```python
from build123d import *

# Parameters (mm, degrees)
CUT_EXTRUDE1_DEPTH = 10
FILLET1_R          = 10
SKETCH5_R          = 2
CUT_EXTRUDE2_DEPTH = 10


with BuildPart() as part:
    # Sketch3 → Revolve1 (revolve)
    with BuildSketch(Plane(origin=(0, 0, 0), x_dir=(0, 0, -1), z_dir=(1, 0, 0))):
        Polygon((0, 12), (7, 12), (7, 8), (17, 8), (17, 12), (24, 12), (24, 35), (19, 35), (19, 17), (0, 17), align=None)
    revolve(axis=Axis((0, 0, 0), (0, 0, -1)))

    # Sketch4 → Cut-Extrude1 (cut)
    with BuildSketch(Plane.XY.offset(-19)):
        with BuildLine():
            ThreePointArc((35, 0), (32.335783638, 13.393920133), (24.748737342, 24.748737342))
            Line((24.748737342, 24.748737342), (24.748737342, -24.748737342))
            ThreePointArc((24.748737342, -24.748737342), (32.335783638, -13.393920133), (35, 0))
        make_face()
        with BuildLine():
            ThreePointArc((24.748737342, 24.748737342), (0, 35), (-24.748737342, 24.748737342))
            Line((-24.748737342, 24.748737342), (24.748737342, 24.748737342))
        make_face()
        with BuildLine():
            Line((-24.748737342, -24.748737342), (-24.748737342, 24.748737342))
            ThreePointArc((-24.748737342, 24.748737342), (-35, 0), (-24.748737342, -24.748737342))
        make_face()
        with BuildLine():
            Line((24.748737342, -24.748737342), (-24.748737342, -24.748737342))
            ThreePointArc((-24.748737342, -24.748737342), (0, -35), (24.748737342, -24.748737342))
        make_face()
    extrude(amount=-CUT_EXTRUDE1_DEPTH, mode=Mode.SUBTRACT)

    # Fillet1
    fillet1_edges = [part.edges().sort_by_distance(p)[0] for p in [
        (24.748737342, 24.748737342, -21.5),
        (24.748737342, -24.748737342, -21.5),
        (-24.748737342, 24.748737342, -21.5),
        (-24.748737342, -24.748737342, -21.5),
    ]]
    fillet(fillet1_edges, radius=FILLET1_R)

    # Sketch5 → Cut-Extrude2 (cut)
    with BuildSketch(Plane(origin=(0, 0, -24), x_dir=(-1, 0, 0), z_dir=(0, 0, -1))):
        with Locations((-17.5, 17.5)):
            Circle(SKETCH5_R)
        with Locations((17.5, 17.5)):
            Circle(SKETCH5_R)
        with Locations((17.5, -17.5)):
            Circle(SKETCH5_R)
        with Locations((-17.5, -17.5)):
            Circle(SKETCH5_R)
    extrude(amount=-CUT_EXTRUDE2_DEPTH, mode=Mode.SUBTRACT)


solid = part.part
```
The listing builds one solid part. Answer for the finished solid, in the listing's coordinates (mm). A direction names the side the tool comes from. Give positions to 0.01 mm unless a question says otherwise; leave off trailing zeros. Order: outer loops, then holes, each group sorted by start corner. A loop starts at its lowest first (then second) coordinate and runs counter-clockwise, first axis right, second up. Notation, with made-up numbers: (-19, -25.75) - (27, -25.75) arc R14 cw to (27, -1.75) - close; hole circle Ø9 at (-11, 57). An arc over 180 degrees is marked (long way). Answer in a Markdown table with one row per item. Add a question column.
Q1. Find the intervals of material crossed by line 1 along Y through (x, z) = (17.5, -20.4); line 2 along X through (y, z) = (15, -10.5); line 3 along Z through (x, y) = (18.5, 14.5), in increasing order. Write a range as [from, to].
Q2. Which of the six approach directions +Z, -Z, +X, -X, +Y, -Y give full straight-line access (tool end or side, diameter ignored) to faces 1 (the flat face through (-8, -2, -17)), 2 (the cylindrical face through (0.53, -11.99, -3.55)), 3 (the cylindrical face through (21.74, -21.9, -21.54))?
Q3. The part is cut by section A-A (x = 0). Determine the outline of the cut face in (y, z), then the cut area to 3 significant figures.
Q4. Given P1, Ø7, axis at x = -4.5, y = -6, coming from the -Z side; P2, Ø2.5, axis at x = 17.5, y = 17.5, coming from the -Z side; P3, Ø10, axis at y = -0.5, z = -4.5, coming from the +X side; P4, Ø2, axis at y = -15.5, z = -13, coming from the +X side, each flat-ended and moving along its own axis, determine where each tip first touches the part or whether it passes through.
Q5. The part is cut by section D-D (z = -8.25). Determine the outline of the cut face in (x, y).
Q6. For a pull along X with two mould halves and no side action, classify faces 4 (the flat face through (6, -17, -19)), 5 (the cylindrical face through (0.53, -11.99, -20.55)), 6 (the flat face through (24.749, 0, -21)) as released by +X, released by -X, zero draft, split by the parting line, or undercut.
Q7. The part is cut by section C-C (z = -22.25). Determine the outline of the cut face in (x, y).
Determined:
| question | item | result |
|---|---|---|
| 1 | line 1 | y = [-24.36, -19.5], [-15.5, 15.5], [19.5, 24.36] |
| 1 | line 2 | x = [-8, 8] |
| 1 | line 3 | z = [-24, -19] |
| 2 | face 1 | -Z |
| 2 | face 2 | +Z |
| 2 | face 3 | +Z, -Z, +X, -Y |
| 3 | outline | (-24.75, -24) - (-12, -24) - (-12, -17) - (-8, -17) - (-8, -7) - (-12, -7) - (-12, 0) - (-17, 0) - (-17, -19) - (-24.75, -19) - close; (8, -17) - (12, -17) - (12, -24) - (24.75, -24) - (24.75, -19) - (17, -19) - (17, 0) - (12, 0) - (12, -7) - (8, -7) - close |
| 3 | area | 397 mm² |
| 4 | P1 | stops at z = -17 |
| 4 | P2 | passes through |
| 4 | P3 | stops at x = 17 |
| 4 | P4 | stops at x = 8.87 |
| 5 | outline | circle Ø34 at (0, 0); hole circle Ø16 at (0, 0) |
| 6 | face 4 | zero draft |
| 6 | face 5 | undercut |
| 6 | face 6 | released by +X |
| 7 | outline | (-24.75, -14.75) arc R10 ccw to (-14.75, -24.75) - (14.75, -24.75) arc R10 ccw to (24.75, -14.75) - (24.75, 14.75) arc R10 ccw to (14.75, 24.75) - (-14.75, 24.75) arc R10 ccw to (-24.75, 14.75) - close; hole circle Ø4 at (-17.5, -17.5); hole circle Ø4 at (-17.5, 17.5); hole circle Ø24 at (0, 0); hole circle Ø4 at (17.5, -17.5); hole circle Ø4 at (17.5, 17.5) |
